The drawing under review shows one solid part. Ordinate dimensions are in mm from its lowest x, y, z. Round coordinates to 2 decimals unless told otherwise and drop trailing zeros. Write each loop counter-clockwise with the first axis right and the second up, starting at its lowest first coordinate (ties: lowest second). Pieces come first, ordered by that corner, then holes.
Item 1: Add section C-C (z = 41). Give the boundary of the cut face in (x, y).
Item 2: Clearance check with flat-ended pins moving along their axes: pin 1 Ø6 at (x, y) = (81.5, 20.5) entering from -Z; pin 2 Ø10.5 at (y, z) = (10.5, 119) entering from -X (1 decimal); pin 3 Ø8 at (x, y) = (74, 10) entering from -Z. State where each tip first meets the part, or that it passes through.
Item 3: Draft analysis for pull direction X (two halves, no side actions). For the marked faces 1, 2, 3 and 4, state which applies: +X half, -X half, draft (parallel to the pull), parting line (faces both ways), or undercut.
Item 4: Add section D-D (x = 27.5). Give the boundary of the cut face in (y, z).
Item 5: Add section A-A (x = 60). Give the boundary of the cut face in (y, z).
Item 6: To check wall thickness, follow L1, parallel to Z at x = 60.5, y = 11.25; L2, parallel to X at y = 9.5, z = 63.5 (1 decimal); L3, parallel to Z at x = 57, y = 14.5 (1 decimal). State the ranges of each line that lie inside material, in increasing order.
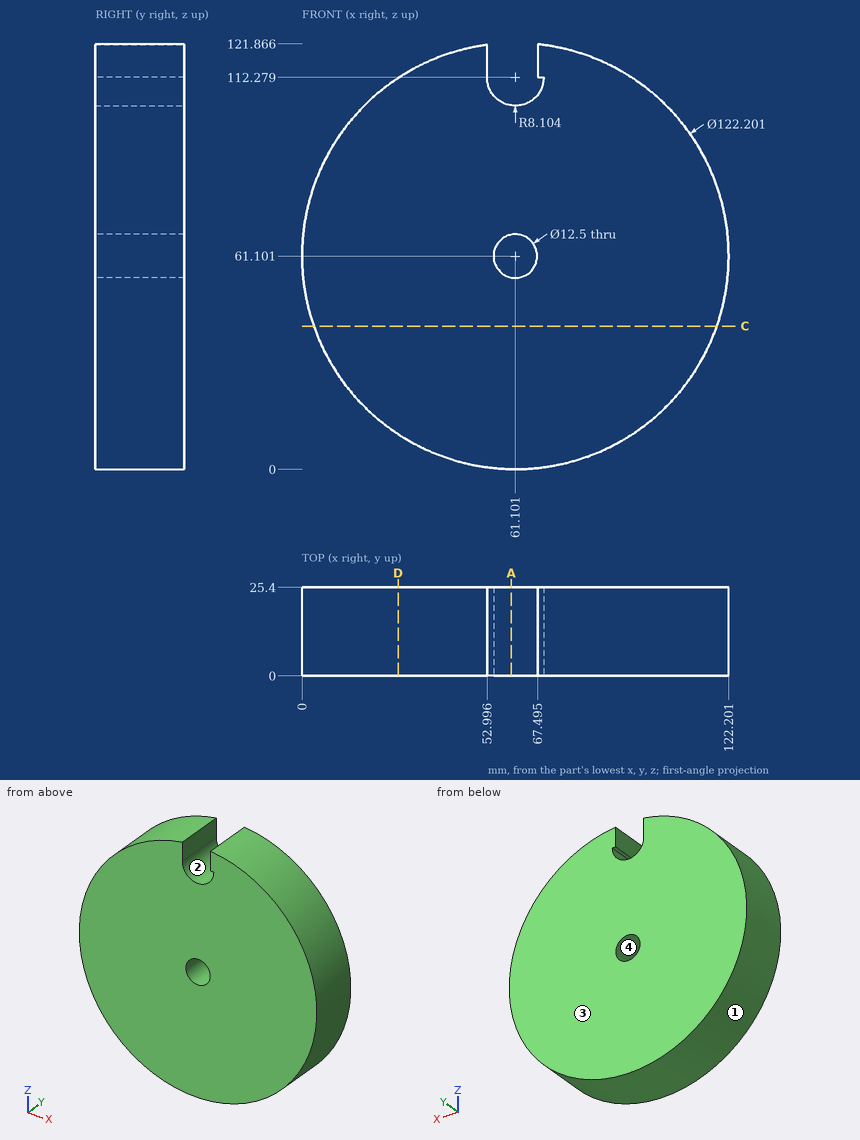
Numbers:
1. outline: (3.4, 0) - (118.8, 0) - (118.8, 25.4) - (3.4, 25.4) - close
2. pin 1: stops at z = 2.53
2. pin 2: stops at x = 30.1
2. pin 3: stops at z = 0.65
3. face 1: parting line
3. face 2: undercut
3. face 3: draft
3. face 4: undercut
4. outline: (0, 10.07) - (25.4, 10.07) - (25.4, 112.13) - (0, 112.13) - close
5. outline: (0, 0.01) - (25.4, 0.01) - (25.4, 54.95) - (0, 54.95) - close; (0, 67.25) - (25.4, 67.25) - (25.4, 104.25) - (0, 104.25) - close
6. L1: z = 0 to 54.88, 67.32 to 104.2
6. L2: x = 0 to 55.3, 66.9 to 122.2
6. L3: z = 0.1 to 56.4, 65.8 to 105.3
